from build123d import *

# Parameters (mm, degrees)
BOSS_EXTRUDE1_DEPTH = 120


with BuildPart() as part:
    # Sketch1 → Boss-Extrude1 (new body, symmetric)
    with BuildSketch(Plane.XY):
        with BuildLine():
            Line((21.799994, 7.139358412), (18.939339529, 9.999998412))
            Line((18.939339529, 9.999998412), (11.060658529, 9.999998412))
            Line((11.060658529, 9.999998412), (8.200003529, 7.139342412))
            Line((8.200003529, 7.139342412), (8.200003529, 2.800001412))
            ThreePointArc((8.200003529, 2.800001412), (8.287868495, 2.58786762), (8.500000529, 2.499998412))
            Line((8.500000529, 2.499998412), (10.400000529, 2.499998412))
            ThreePointArc((10.400000529, 2.499998412), (10.75355392, 2.353551802), (10.900000529, 1.999998412))
            Line((10.900000529, 1.999998412), (10.900000529, 0.299995529))
            ThreePointArc((10.900000529, 0.299995529), (10.812133796, 0.08786744), (10.600006, 0))
            Line((10.600006, 0), (2.5, 0))
            ThreePointArc((2.5, 0), (0.732233047, 0.732233047), (0, 2.5))
            Line((0, 2.5), (0, 10.600006))
            ThreePointArc((0, 10.600006), (0.087869562, 10.812137388), (0.300003, 10.900002))
            Line((0.300003, 10.900002), (2, 10.900002))
            ThreePointArc((2, 10.900002), (2.353553391, 10.753555391), (2.5, 10.400002))
            Line((2.5, 10.400002), (2.5, 8.500002))
            ThreePointArc((2.5, 8.500002), (2.587869099, 8.287870075), (2.80000269, 8.200005))
            Line((2.80000269, 8.200005), (7.139344, 8.200005))
            Line((7.139344, 8.200005), (10, 11.06066))
            Line((10, 11.06066), (10, 18.939341))
            Line((10, 18.939341), (7.139344, 21.799985148))
            Line((7.139344, 21.799985148), (2.800003, 21.799985148))
            ThreePointArc((2.800003, 21.799985148), (2.587872691, 21.712123666), (2.5, 21.499998))
            Line((2.5, 21.499998), (2.5, 19.599988398))
            ThreePointArc((2.5, 19.599988398), (2.353553317, 19.246434831), (1.99999975, 19.099988148))
            Line((1.99999975, 19.099988148), (0.299996735, 19.099988148))
            ThreePointArc((0.299996735, 19.099988148), (0.0878677, 19.187854622), (0, 19.399983148))
            Line((0, 19.399983148), (0, 27.499989148))
            ThreePointArc((0, 27.499989148), (0.732232787, 29.267756841), (2.500000265, 29.999990148))
            Line((2.500000265, 29.999990148), (10.6000062, 29.999990148))
            ThreePointArc((10.6000062, 29.999990148), (10.812133482, 29.912123021), (10.900000529, 29.699995706))
            Line((10.900000529, 29.699995706), (10.900000529, 27.999998706))
            ThreePointArc((10.900000529, 27.999998706), (10.753556384, 27.64644081), (10.400000529, 27.499991736))
            Line((10.400000529, 27.499991736), (8.499998529, 27.499991736))
            ThreePointArc((8.499998529, 27.499991736), (8.287867897, 27.41212193), (8.200003529, 27.199989046))
            Line((8.200003529, 27.199989046), (8.200003529, 22.860646736))
            Line((8.200003529, 22.860646736), (11.060659, 19.999991736))
            Line((11.060659, 19.999991736), (18.93934, 19.999991736))
            Line((18.93934, 19.999991736), (21.799994, 22.860646736))
            Line((21.799994, 22.860646736), (21.799994, 27.199988736))
            ThreePointArc((21.799994, 27.199988736), (21.712128868, 27.412122694), (21.499996529, 27.499991736))
            Line((21.499996529, 27.499991736), (19.599998, 27.499991736))
            ThreePointArc((19.599998, 27.499991736), (19.246444609, 27.646438346), (19.099998, 27.999991736))
            Line((19.099998, 27.999991736), (19.099998, 29.700007823))
            ThreePointArc((19.099998, 29.700007823), (19.187864526, 29.912137383), (19.3999935, 30.000005323))
            Line((19.3999935, 30.000005323), (27.4999995, 30.000005323))
            ThreePointArc((27.4999995, 30.000005323), (29.267773609, 29.267772326), (30.000009773, 27.499999529))
            Line((30.000009773, 27.499999529), (30.000009773, 19.399993594))
            ThreePointArc((30.000009773, 19.399993594), (29.912139919, 19.187852468), (29.6999965, 19.099988148))
            Line((29.6999965, 19.099988148), (27.9999995, 19.099988148))
            ThreePointArc((27.9999995, 19.099988148), (27.64645275, 19.246438389), (27.500009772, 19.599988147))
            Line((27.500009772, 19.599988147), (27.500009772, 21.499990147))
            ThreePointArc((27.500009772, 21.499990147), (27.412139967, 21.712120779), (27.200007083, 21.799985148))
            Line((27.200007083, 21.799985148), (22.860664773, 21.799985148))
            Line((22.860664773, 21.799985148), (20.000009773, 18.939341))
            Line((20.000009773, 18.939341), (20.000009773, 11.06066))
            Line((20.000009773, 11.06066), (22.8606545, 8.200005))
            Line((22.8606545, 8.200005), (27.1999965, 8.200005))
            ThreePointArc((27.1999965, 8.200005), (27.412129602, 8.287869277), (27.499999499, 8.500000052))
            Line((27.499999499, 8.500000052), (27.499999499, 10.400002001))
            ThreePointArc((27.499999499, 10.400002001), (27.646446109, 10.753555391), (27.9999995, 10.900002))
            Line((27.9999995, 10.900002), (29.7000025, 10.900002))
            ThreePointArc((29.7000025, 10.900002), (29.912138814, 10.812138492), (30.000009773, 10.600005265))
            Line((30.000009773, 10.600005265), (30.000009773, 2.499999265))
            ThreePointArc((30.000009773, 2.499999265), (29.267773942, 0.732224081), (27.500000177, -1.5175e-05))
            Line((27.500000177, -1.5175e-05), (19.399994245, -1.5175e-05))
            ThreePointArc((19.399994245, -1.5175e-05), (19.187855627, 0.08786137), (19.099998, 0.300007824))
            Line((19.099998, 0.300007824), (19.099998, 2.000004824))
            ThreePointArc((19.099998, 2.000004824), (19.246446356, 2.353553549), (19.599996529, 2.499998412))
            Line((19.599996529, 2.499998412), (21.499998529, 2.499998412))
            ThreePointArc((21.499998529, 2.499998412), (21.712135123, 2.587873708), (21.799994, 2.800017102))
            Line((21.799994, 2.800017102), (21.799994, 7.139358412))
        make_face()
        with BuildLine():
            Line((18.878868942, 11.714100014), (18.657285002, 12.75690673))
            Line((18.657285002, 12.75690673), (18.419345869, 12.994846743))
            ThreePointArc((18.419345869, 12.994846743), (18.335473622, 13.158180995), (18.362480424, 13.339793948))
            ThreePointArc((18.362480424, 13.339793948), (18.750006156, 14.99998656), (18.362487962, 16.660180933))
            ThreePointArc((18.362487962, 16.660180933), (18.335481889, 16.841794157), (18.419354758, 17.005128271))
            Line((18.419354758, 17.005128271), (18.657294593, 17.243067582))
            Line((18.657294593, 17.243067582), (18.878893628, 18.28587109))
            ThreePointArc((18.878893628, 18.28587109), (18.743367928, 18.743355263), (18.285883756, 18.878880962))
            Line((18.285883756, 18.878880962), (17.243080247, 18.657281928))
            Line((17.243080247, 18.657281928), (17.005140412, 18.419342617))
            ThreePointArc((17.005140412, 18.419342617), (16.84180664, 18.335470316), (16.660194009, 18.362476539))
            ThreePointArc((16.660194009, 18.362476539), (15.00000526, 18.749996344), (13.339816433, 18.362476869))
            ThreePointArc((13.339816433, 18.362476869), (13.158203164, 18.335470716), (12.994869031, 18.419343671))
            Line((12.994869031, 18.419343671), (12.756929898, 18.657283684))
            Line((12.756929898, 18.657283684), (11.714126233, 18.878881984))
            ThreePointArc((11.714126233, 18.878881984), (11.256641967, 18.743355772), (11.121116891, 18.28587117))
            Line((11.121116891, 18.28587117), (11.342717777, 17.243068055))
            Line((11.342717777, 17.243068055), (11.580656587, 17.00512772))
            ThreePointArc((11.580656587, 17.00512772), (11.664528478, 16.841794182), (11.637522309, 16.660181943))
            ThreePointArc((11.637522309, 16.660181943), (11.250003617, 14.999998075), (11.637519652, 13.339813587))
            ThreePointArc((11.637519652, 13.339813587), (11.664525497, 13.15820068), (11.580652734, 12.994866901))
            Line((11.580652734, 12.994866901), (11.342712898, 12.75692759))
            Line((11.342712898, 12.75692759), (11.12111194, 11.71412449))
            ThreePointArc((11.12111194, 11.71412449), (11.256636795, 11.256640068), (11.714120718, 11.121113524))
            Line((11.714120718, 11.121113524), (12.756924635, 11.342710635))
            Line((12.756924635, 11.342710635), (12.99486447, 11.580649946))
            ThreePointArc((12.99486447, 11.580649946), (13.158198441, 11.66452228), (13.339811235, 11.637515845))
            ThreePointArc((13.339811235, 11.637515845), (14.999988879, 11.249993804), (16.660169832, 11.637501672))
            ThreePointArc((16.660169832, 11.637501672), (16.841782614, 11.664506717), (17.005115943, 11.580633605))
            Line((17.005115943, 11.580633605), (17.243054753, 11.34269327))
            Line((17.243054753, 11.34269327), (18.285858839, 11.12109695))
            ThreePointArc((18.285858839, 11.12109695), (18.743339639, 11.256620822), (18.878868942, 11.714100014))
        make_face(mode=Mode.SUBTRACT)
        with BuildLine():
            Line((23.299995, 1), (27.5, 1))
            ThreePointArc((27.5, 1), (28.56065669, 1.439341852), (28.999994597, 2.500000176))
            Line((28.999994597, 2.500000176), (28.999994597, 6.700005176))
            ThreePointArc((28.999994597, 6.700005176), (28.853547926, 7.053558453), (28.499994597, 7.200005))
            Line((28.499994597, 7.200005), (24.299995, 7.200005))
            ThreePointArc((24.299995, 7.200005), (23.239334828, 6.760665172), (22.799995, 5.700005))
            Line((22.799995, 5.700005), (22.799995, 1.5))
            ThreePointArc((22.799995, 1.5), (22.946441609, 1.146446609), (23.299995, 1))
        make_face(mode=Mode.SUBTRACT)
        with BuildLine():
            Line((2.5, 1), (6.700005, 1))
            ThreePointArc((6.700005, 1), (7.05355839, 1.146446609), (7.200005, 1.5))
            Line((7.200005, 1.5), (7.200005, 5.700005))
            ThreePointArc((7.200005, 5.700005), (6.760665172, 6.760665172), (5.700005, 7.200005))
            Line((5.700005, 7.200005), (1.5, 7.200005))
            ThreePointArc((1.5, 7.200005), (1.146446609, 7.053558391), (1, 6.700005))
            Line((1, 6.700005), (1, 2.5))
            ThreePointArc((1, 2.5), (1.439339828, 1.439339828), (2.5, 1))
        make_face(mode=Mode.SUBTRACT)
        with BuildLine():
            Line((1.5, 22.799985148), (5.700005, 22.799985148))
            ThreePointArc((5.700005, 22.799985148), (6.760665172, 23.239324976), (7.200005, 24.299985148))
            Line((7.200005, 24.299985148), (7.200005, 28.499990148))
            ThreePointArc((7.200005, 28.499990148), (7.053558391, 28.853543539), (6.700005, 28.999990148))
            Line((6.700005, 28.999990148), (2.5, 28.999990148))
            ThreePointArc((2.5, 28.999990148), (1.439339828, 28.56065032), (1, 27.499990148))
            Line((1, 27.499990148), (1, 23.299985148))
            ThreePointArc((1, 23.299985148), (1.146446609, 22.946431757), (1.5, 22.799985148))
        make_face(mode=Mode.SUBTRACT)
        with BuildLine():
            Line((24.299995, 22.799985148), (28.499994597, 22.799985148))
            ThreePointArc((28.499994597, 22.799985148), (28.853551502, 22.946435272), (28.999994597, 23.299995088))
            Line((28.999994597, 23.299995088), (28.999994597, 27.500000088))
            ThreePointArc((28.999994597, 27.500000088), (28.560656076, 28.560654835), (27.5, 28.999990148))
            Line((27.5, 28.999990148), (23.299995, 28.999990148))
            ThreePointArc((23.299995, 28.999990148), (22.94644161, 28.853543539), (22.799995, 28.499990148))
            Line((22.799995, 28.499990148), (22.799995, 24.299985148))
            ThreePointArc((22.799995, 24.299985148), (23.239334828, 23.239324976), (24.299995, 22.799985148))
        make_face(mode=Mode.SUBTRACT)
    extrude(amount=BOSS_EXTRUDE1_DEPTH, both=True)


solid = part.part
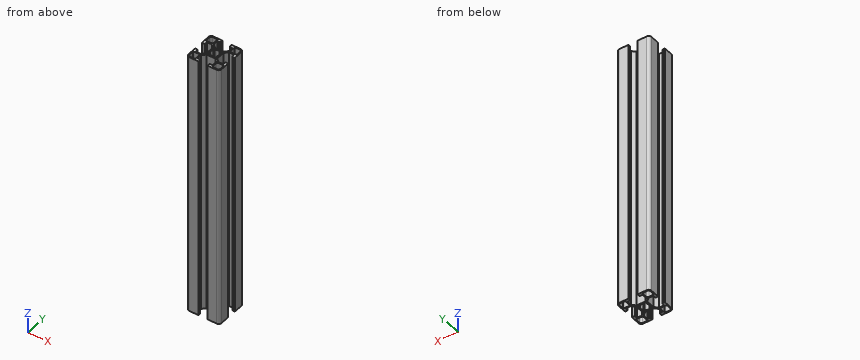
The model under review builds one solid part; all positions refer to its coordinate system, in mm. Coordinates: 2 decimals unless noted, no trailing zeros. Answer in a Markdown table with one row per item.
1. Wall thickness on probe 1 along X at (y, z) = (24, -103.5); probe 2 along Y at (x, z) = (26, 97); probe 3 along X at (y, z) = (21, 78.5): over which ranges is each line inside the solid? List them lowest first. Write a range as [from, to].
Answers below:
| item | result |
|---|---|
| probe 1 | x = [0, 1], [7.17, 8.2], [21.8, 22.83], [29, 30] |
| probe 2 | y = [0, 1], [7.2, 8.2], [21.8, 22.8], [29, 30] |
| probe 3 | x = [0, 2.5], [7.94, 10.06], [19.94, 22.06], [27.5, 30] |
2. We need section A-A, the plane z = -11.5. Give the number of separate pieces and of enclosed holes in the cut face, and give its area (3 significant figures).
Answers below:
| item | result |
|---|---|
| separate pieces | 1 |
| enclosed holes | 5 |
| area | 234 mm^2 |
3. Clearance check with flat-ended pins moving along their axes: pin 1 Ø1.4 at (y, z) = (29, 46) entering from +X; pin 2 Ø0.9 at (y, z) = (29, 21) entering from -X; pin 3 Ø1.4 at (y, z) = (1.5, -55.5) entering from -X. State where each tip first meets the part, or that it passes through.
Answers below:
| item | result |
|---|---|
| pin 1 | stops at x = 29.87 |
| pin 2 | stops at x = 0.23 |
| pin 3 | stops at x = 0.02 |
